```python
from build123d import *

# Parameters (mm, degrees)
SKETCH027_W   = 68
SKETCH027_H   = 36
PAD015_DEPTH  = 1
SKETCH028_W   = 68
SKETCH028_H   = 36
SKETCH028_W_2 = 66
SKETCH028_H_2 = 34
PAD016_DEPTH  = 3
SKETCH029_W   = 3.04
SKETCH029_H   = 13.335
PAD017_DEPTH  = 3
SKETCH032_R   = 1.5
PAD020_DEPTH  = 3
BOX_W         = 70
BOX_H         = 38
BOX_DEPTH     = 5


with BuildPart() as topmold:
    # Sketch027 → Pad015 (new body)
    with BuildSketch(Plane.XY):
        Rectangle(SKETCH027_W, SKETCH027_H)
    extrude(amount=PAD015_DEPTH)

    # Sketch028 (on Face6 of Pad015) → Pad016 (join)
    with BuildSketch(Plane.XY.offset(1)):
        Rectangle(SKETCH028_W, SKETCH028_H)
        Rectangle(SKETCH028_W_2, SKETCH028_H_2, mode=Mode.SUBTRACT)
    extrude(amount=PAD016_DEPTH)

    # Sketch029 (on Face15 of Pad016) → Pad017 (join)
    with BuildSketch(Plane.XY.offset(1)):
        with Locations((-24.94, 4.5625)):
            Rectangle(SKETCH029_W, SKETCH029_H)
    extrude(amount=PAD017_DEPTH)

    # Sketch032 (on Face15 of Pad017) → Pad020 (join)
    with BuildSketch(Plane.XY.offset(1)):
        with Locations((-31, 15)):
            Circle(SKETCH032_R)
        with Locations((31, 15)):
            Circle(SKETCH032_R)
        with Locations((-31, -15)):
            Circle(SKETCH032_R)
        with Locations((31, -15)):
            Circle(SKETCH032_R)
    extrude(amount=PAD020_DEPTH)


with BuildPart() as topmold_1:
    # Body005 placement: moved
    add(topmold.part.moved(Location((100, 39, 0))))


with BuildPart() as top_mold:
    # Box → Box (new body)
    with BuildSketch(Plane(origin=(65, 20, 0), x_dir=(1, 0, 0), z_dir=(0, 0, 1))):
        with Locations((35, 19)):
            Rectangle(BOX_W, BOX_H)
    extrude(amount=BOX_DEPTH)

    # Cut: cut TopMold
    add(topmold_1.part, mode=Mode.SUBTRACT)


solid = top_mold.part
```
Work out the finished part from the listing and answer in its coordinate system (mm). A direction names the side the tool comes from. Give positions to 0.01 mm unless a question says otherwise; leave off trailing zeros. Order: outer loops, then holes, each group sorted by start corner. A loop starts at its lowest first (then second) coordinate and runs counter-clockwise, first axis right, second up. Notation, with made-up numbers: M 47.25,0.25 L 73.25,0.25 A37 ccw 73.25,37.25 Z; hole C 84.5,48 d1. An arc over 180 degrees is marked long. Return JSON: item names as keys, results as strings.
1) Section A-A, the plane z = 1.75 is taken. Write down the section's boundary in (x, y) (3 decimals).
Resolved:
{"outline": "M 65,20 L 135,20 L 135,58 L 65,58 Z; M 67,22 L 133,22 L 133,56 L 67,56 Z; hole M 66,21 L 134,21 L 134,57 L 66,57 Z; hole C 69,24 d3; hole C 69,54 d3; hole M 73.54,36.895 L 76.58,36.895 L 76.58,50.23 L 73.54,50.23 Z; hole C 131,24 d3; hole C 131,54 d3"}
2) Section C-C, the plane x = 69 is taken. Write down the section's boundary in (y, z).
Resolved:
{"outline": "M 20,0 L 21,0 L 21,4 L 22,4 L 22,1 L 22.5,1 L 22.5,4 L 25.5,4 L 25.5,1 L 52.5,1 L 52.5,4 L 55.5,4 L 55.5,1 L 56,1 L 56,4 L 57,4 L 57,0 L 58,0 L 58,5 L 20,5 Z"}
3) Section B-B, the plane y = 24 is taken. Write down the section's boundary in (x, z), plus the area to 3 significant figures.
Resolved:
{"outline": "M 65,0 L 66,0 L 66,4 L 67,4 L 67,1 L 67.5,1 L 67.5,4 L 70.5,4 L 70.5,1 L 129.5,1 L 129.5,4 L 132.5,4 L 132.5,1 L 133,1 L 133,4 L 134,4 L 134,0 L 135,0 L 135,5 L 65,5 Z", "area": "258 mm^2"}
4) Section D-D, the plane y = 31.5 is taken. Write down the section's boundary in (x, z).
Resolved:
{"outline": "M 65,0 L 66,0 L 66,4 L 67,4 L 67,1 L 133,1 L 133,4 L 134,4 L 134,0 L 135,0 L 135,5 L 65,5 Z"}
5) For a pull along Y with two mould halves and no side action, classify faces 3 (the flat face through (100, 58, 2)), 4 (the flat face through (100, 57, 2)), 5 (the flat face through (65, 39, 2)) as +Y half, -Y half, draft (parallel to the pull), parting line (faces both ways), or undercut.
Resolved:
{"face 3": "+Y half", "face 4": "undercut", "face 5": "draft"}
6) A tool of negligible diameter and unlimited length cuts with its end or side. For faces 1 (the flat face through (133, 39, 2)), 2 (the flat face through (135, 39, 2)), from which of +Z, -Z, +X, -X, +Y, -Y can it reach the whole face along a straight path? Write none if from no direction.
Resolved:
{"face 1": "-Z", "face 2": "+Z, -Z, +X, +Y, -Y"}
7) Straight lines are drawn through the part: line 1 along Y through (x, z) = (100.5, 1.35); line 2 along Y through (x, z) = (131, 1.7); line 3 along X through (y, z) = (30, 3.2). For each, find the intervals that lie inside material, in ascending order. Write a range as [from, to].
Resolved:
{"line 1": "[20, 21], [22, 56], [57, 58]", "line 2": "[20, 21], [22, 22.5], [25.5, 52.5], [55.5, 56], [57, 58]", "line 3": "[65, 66], [67, 133], [134, 135]"}
8) Each of these flat-tipped pins is pushed along its axis until it touches: pin 1 (3.5 mm diameter, centred on x = 75.5, y = 46, fed in from -Z); pin 2 (1.5 mm diameter, centred on x = 130.5, y = 53.5, fed in from -Z). Where does it stop, or does it pass through?
Resolved:
{"pin 1": "z = 1", "pin 2": "z = 4"}
